```python
from build123d import *

# Parameters (mm, degrees)
SKETCH1_R           = 35.5981
BOSS_EXTRUDE1_DEPTH = 13.5128
SKETCH2_R           = 25.2095
CUT_EXTRUDE1_DEPTH  = 40.64
FILLET1_R           = 0.381
FILLET2_R           = 0.381
CHAMFER1_SIZE       = 1.2573
CHAMFER2_SIZE       = 1.2573


with BuildPart() as part:
    # Sketch1 → Boss-Extrude1 (new body)
    with BuildSketch(Plane(origin=(0, 0, 0), x_dir=(1, 0, 0), z_dir=(0, 1, 0))):
        Circle(SKETCH1_R)
    extrude(amount=BOSS_EXTRUDE1_DEPTH)

    # Sketch2 → Cut-Extrude1 (cut)
    with BuildSketch(Plane(origin=(0, 13.5128, 0), x_dir=(1, 0, 0), z_dir=(0, 1, 0))):
        Circle(SKETCH2_R)
    extrude(amount=-CUT_EXTRUDE1_DEPTH, mode=Mode.SUBTRACT)

    # Fillet1
    fillet1_edges = [part.edges().sort_by_distance(p)[0] for p in [
        (-35.5981, 13.5128, 0),
    ]]
    fillet(fillet1_edges, radius=FILLET1_R)

    # Fillet2
    fillet2_edges = [part.edges().sort_by_distance(p)[0] for p in [
        (-35.5981, 0, 0),
    ]]
    fillet(fillet2_edges, radius=FILLET2_R)

    # Chamfer1
    chamfer1_edges = [part.edges().sort_by_distance(p)[0] for p in [
        (-25.2095, 13.5128, 0),
    ]]
    chamfer(chamfer1_edges, length=CHAMFER1_SIZE)

    # Chamfer2
    chamfer2_edges = [part.edges().sort_by_distance(p)[0] for p in [
        (-25.2095, 0, 0),
    ]]
    chamfer(chamfer2_edges, length=CHAMFER2_SIZE)


solid = part.part
```
CAD build for the part. Positions are in the model's coordinates, mm. Coordinates: 2 decimals unless noted, no trailing zeros. Order: outer loops, then holes, each group sorted by start corner. A loop starts at its lowest first (then second) coordinate and runs counter-clockwise, first axis right, second up. Notation, with made-up numbers: M 81.5,-22.5 L 104.5,-22.5 A28 cw 104.5,6.5 Z; hole C 41.25,73 d9. An arc over 180 degrees is marked long. Answer as CSV lines item,"result".
1) Mould opens along X. For faces 1 (the flat face through (5.1, 0, -26.3)), 2 (the cylindrical face through (-7.72, 6.67, 34.75)), 3 (the cylindrical face through (-25.185, 6.833, -1.108)) say: released by +X, released by -X, zero draft, split by the parting line, or undercut.
Verdict:
face 1,"zero draft"
face 2,"split by the parting line"
face 3,"undercut"
2) Cut at B-B (x = 0). List the corners of the cut face in (y, z), then the cut area to 3 significant figures.
Verdict:
outline,"M 0,-35.22 A0.38 ccw 0.38,-35.6 L 13.13,-35.6 A0.38 ccw 13.51,-35.22 L 13.51,-26.47 L 12.26,-25.21 L 1.26,-25.21 L 0,-26.47 Z; M 0,26.47 L 1.26,25.21 L 12.26,25.21 L 13.51,26.47 L 13.51,35.22 A0.38 ccw 13.13,35.6 L 0.38,35.6 A0.38 ccw 0,35.22 Z"
area,"277 mm2"
3) Flat gauge pins, fed straight in: P1, Ø1, axis at y = 6.5, z = -4.5, coming from the -X side; P2, Ø12, axis at x = 22, z = -7, coming from the -Y side; P3, Ø5, axis at x = 24.5, y = 10, coming from the +Z side; P4, Ø1, axis at x = 15, y = 6, coming from the -Z side. Where does each tip first touch, or does it go through?
Verdict:
P1,"x = -35.37"
P2,"y = 0"
P3,"z = 27.99"
P4,"z = -32.51"
4) Cut at A-A (z = 0). List the corners of the cut face in (x, y).
Verdict:
outline,"M -35.6,0.38 A0.38 ccw -35.22,0 L -26.47,0 L -25.21,1.26 L -25.21,12.26 L -26.47,13.51 L -35.22,13.51 A0.38 ccw -35.6,13.13 Z; M 25.21,1.26 L 26.47,0 L 35.22,0 A0.38 ccw 35.6,0.38 L 35.6,13.13 A0.38 ccw 35.22,13.51 L 26.47,13.51 L 25.21,12.26 Z"
5) Cut at C-C (y = 7.75). List the corners of the cut face in (x, z), then the cut area to 3 significant figures.
Verdict:
outline,"C 0,0 d71.2; hole C 0,0 d50.42"
area,"1,980 mm2"
6) Drill centre lines: L1, parallel to Z at x = 0, y = 8.25; L2, parallel to Z at x = 7.5, y = 7.75. Where is each one in solid material? Low to high. Write a range as from..to.
Verdict:
L1,"-35.6..-25.21, 25.21..35.6"
L2,"-34.8..-24.07, 24.07..34.8"
